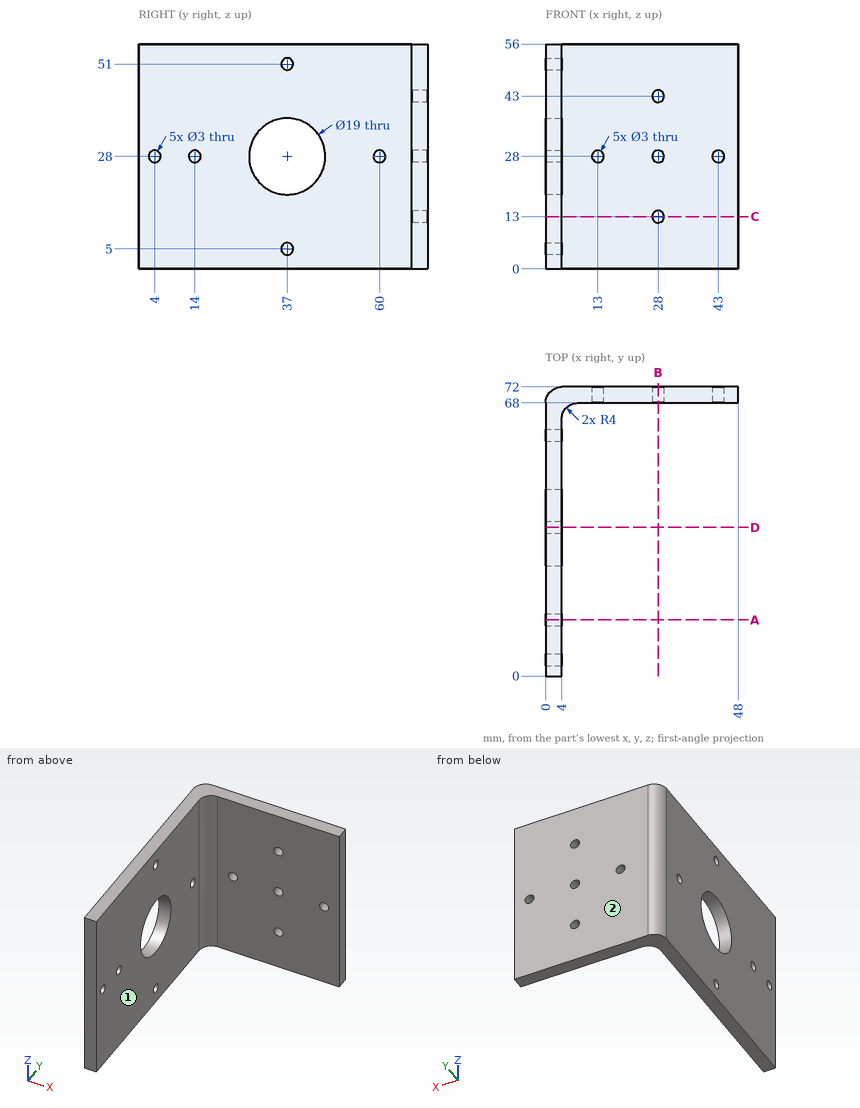
Geometry check sheet. Reference: drawing and pictorial views, mm from the part's lowest x, y, z. A direction names the side the tool comes from. Coordinates: 2 decimals unless noted, no trailing zeros. Order: outer loops, then holes, each group sorted by start corner. A loop starts at its lowest first (then second) coordinate and runs counter-clockwise, first axis right, second up. Notation, with made-up numbers: (-24, 43) - (-9, 43) arc R24 cw to (-9, 65) - close; hole circle Ø6 at (40, 29). An arc over 180 degrees is marked (long way). Answer in a Markdown table with one row per item. Add a question column.
1) Cross-section at B-B, the plane x = 28. Record the cut outline in (y, z), then the cut area to 3 significant figures.
2) Cross-section at A-A, the plane y = 14. Record the cut outline in (x, z).
3) Cross-section at D-D, the plane y = 37. Record the cut outline in (x, z).
4) Gauge pin test, flat ends, axial feed: P1, Ø3.5, axis at y = 37, z = 51, coming from the -X side; P2, Ø4, axis at x = 38, z = 34.5, coming from the -Y side; P3, Ø3.5, axis at y = 14, z = 28, coming from the +X side. Record the tip position at first contact, or that the pin passes through.
5) Set-up check for the marked faces 1 and 2: record each of +Z, -Z, +X, -X, +Y, -Y from which the full face is reachable in a straight line by a thin tool's end or side.
6) Cross-section at C-C, the plane z = 13. Record the cut outline in (x, y).
7) Material ranges on line 1 along X through (y, z) = (22, 51); line 2 along Y through (x, z) = (42.5, 53.5); line 3 along Y through (x, z) = (2, 51), recorded low to high. Write a range as [from, to].
Check result:
| question | item | result |
|---|---|---|
| 1 | outline | (68, 0) - (72, 0) - (72, 11.5) - (68, 11.5) - close; (68, 14.5) - (72, 14.5) - (72, 26.5) - (68, 26.5) - close; (68, 29.5) - (72, 29.5) - (72, 41.5) - (68, 41.5) - close; (68, 44.5) - (72, 44.5) - (72, 56) - (68, 56) - close |
| 1 | area | 188 mm² |
| 2 | outline | (0, 0) - (4, 0) - (4, 26.5) - (0, 26.5) - close; (0, 29.5) - (4, 29.5) - (4, 56) - (0, 56) - close |
| 3 | outline | (0, 0) - (4, 0) - (4, 3.5) - (0, 3.5) - close; (0, 6.5) - (4, 6.5) - (4, 18.5) - (0, 18.5) - close; (0, 37.5) - (4, 37.5) - (4, 49.5) - (0, 49.5) - close; (0, 52.5) - (4, 52.5) - (4, 56) - (0, 56) - close |
| 4 | P1 | stops at x = 0 |
| 4 | P2 | stops at y = 68 |
| 4 | P3 | stops at x = 4 |
| 5 | face 1 | +Z, -Z, +X, -Y |
| 5 | face 2 | +Z, -Z, +X, -X, +Y |
| 6 | outline | (0, 0) - (4, 0) - (4, 64) arc R4 cw to (8, 68) - (26.5, 68) - (26.5, 72) - (4, 72) arc R4 ccw to (0, 68) - close; (29.5, 68) - (48, 68) - (48, 72) - (29.5, 72) - close |
| 7 | line 1 | x = [0, 4] |
| 7 | line 2 | y = [68, 72] |
| 7 | line 3 | y = [0, 35.5], [38.5, 71.46] |
